Check sheet for the modelled part. Datum: model origin and axes. Units: mm. A direction names the side the tool comes from. Give positions to 0.01 mm unless a question says otherwise; leave off trailing zeros. Order: outer loops, then holes, each group sorted by start corner. A loop starts at its lowest first (then second) coordinate and runs counter-clockwise, first axis right, second up. Notation, with made-up numbers: (3.5, 45.5) -> (18.5, 45.5) arc R16 ccw to (18.5, 66.5) -> close; hole circle Ø10 at (60, -13). An arc over 180 degrees is marked (long way). Answer in a Markdown table with one row per item. Add a question column.
(1) Cross-section at B-B (z = 0). Record the cut outline in (x, y), then the cut area to 3 significant figures.
(2) Go/stop test with flat-tipped pins: pin 1 (2 mm diameter, centred on y = 20, z = -5, fed in from +X); pin 2 (3 mm diameter, centred on x = -19.5, z = -0.5, fed in from -Y); pin 3 (1.5 mm diameter, centred on y = 30.5, z = 3, fed in from +X). Record where each tip stops, or that it passes through.
(3) Cross-section at A-A (y = 4.5). Record the cut outline in (x, z).
(4) Thickness scan on L1, parallel to X at y = 13, z = 4.5; L2, parallel to Y at x = 23, z = 0. Record the ranges inside material, lowest first. Write a range as [from, to].
(5) Cross-section at D-D (y = 30). Record the cut outline in (x, z), then the cut area to 3 significant figures.
(6) Release check for a two-part mould opening along X. For faces 1 (the face through (0, 8, -12.7)), 2 (the face through (-25.4, 19, 0)), 3 (the face through (-2.86, 28.36, -5.22)) record: released by +X, released by -X, zero draft, split by the parting line, or undercut.
(7) Set-up check for faces 4 (the face through (-12.7, 8, 0)), 5 (the face through (-3, 31.4, 0)), 6 (the face through (22.269, 36.109, -6.827)): record each of +Z, -Z, +X, -X, +Y, -Y from which the full face is reachable in a straight line by a thin tool's end or side.
(8) Cross-section at C-C (x = 16.5). Record the cut outline in (y, z).
```python
from build123d import *

# Parameters (mm, degrees)
SKETCH2_W           = 50.8
SKETCH2_H           = 50.8
BOSS_EXTRUDE1_DEPTH = 50.8
SKETCH3_W           = 25.4
SKETCH3_H           = 25.4
SKETCH3_W_2         = 22.352
SKETCH3_H_2         = 22.352
CUT_EXTRUDE1_DEPTH  = 15.24
CUT_EXTRUDE2_DEPTH  = 51.8
SKETCH5_R           = 12.7
CUT_EXTRUDE3_DEPTH  = 6.35


with BuildPart() as part:
    # Sketch2 → Boss-Extrude1 (new body)
    with BuildSketch(Plane(origin=(0, 0, 0), x_dir=(1, 0, 0), z_dir=(0, 1, 0))):
        Rectangle(SKETCH2_W, SKETCH2_H)
    extrude(amount=BOSS_EXTRUDE1_DEPTH)

    # Sketch3 → Cut-Extrude1 (cut)
    with BuildSketch(Plane.XZ):
        Rectangle(SKETCH3_W, SKETCH3_H)
        Rectangle(SKETCH3_W_2, SKETCH3_H_2, mode=Mode.SUBTRACT)
    extrude(amount=-CUT_EXTRUDE1_DEPTH, mode=Mode.SUBTRACT)

    # Sketch4 → Cut-Extrude2 (cut, through all)
    with BuildSketch(Plane(origin=(25.4, 0, 0), x_dir=(0, 0, -1), z_dir=(1, 0, 0))):
        Polygon((6.92820323, 25.4), (3.464101615, 31.4), (-3.464101615, 31.4), (-6.92820323, 25.4), (-3.464101615, 19.4), (3.464101615, 19.4), align=None)
    extrude(amount=-CUT_EXTRUDE2_DEPTH, mode=Mode.SUBTRACT)

    # Sketch5 → Cut-Extrude3 (cut)
    with BuildSketch(Plane(origin=(25.4, 0, 0), x_dir=(0, 0, -1), z_dir=(1, 0, 0))):
        with Locations((0, 25.4)):
            Circle(SKETCH5_R)
    extrude(amount=-CUT_EXTRUDE3_DEPTH, mode=Mode.SUBTRACT)


solid = part.part
```
Answer below:
| question | item | result |
|---|---|---|
| 1 | outline | (-25.4, 0) -> (-12.7, 0) -> (-12.7, 15.24) -> (-11.18, 15.24) -> (-11.18, 0) -> (11.18, 0) -> (11.18, 15.24) -> (12.7, 15.24) -> (12.7, 0) -> (25.4, 0) -> (25.4, 12.7) -> (19.05, 12.7) -> (19.05, 19.4) -> (-25.4, 19.4) -> close; (-25.4, 31.4) -> (19.05, 31.4) -> (19.05, 38.1) -> (25.4, 38.1) -> (25.4, 50.8) -> (-25.4, 50.8) -> close |
| 1 | area | 1,840 mm² |
| 2 | pin 1 | stops at x = 19.05 |
| 2 | pin 2 | stops at y = 0 |
| 2 | pin 3 | passes through |
| 3 | outline | (-25.4, -25.4) -> (25.4, -25.4) -> (25.4, 25.4) -> (-25.4, 25.4) -> close; (-11.18, -11.18) -> (11.18, -11.18) -> (11.18, 11.18) -> (-11.18, 11.18) -> close; hole (-12.7, -12.7) -> (12.7, -12.7) -> (12.7, 12.7) -> (-12.7, 12.7) -> close |
| 4 | L1 | x = [-25.4, -12.7], [-11.18, 11.18], [12.7, 25.4] |
| 4 | L2 | y = [0, 12.7], [38.1, 50.8] |
| 5 | outline | (-25.4, -25.4) -> (25.4, -25.4) -> (25.4, -11.84) -> (19.05, -11.84) -> (19.05, -4.27) -> (-25.4, -4.27) -> close; (-25.4, 4.27) -> (19.05, 4.27) -> (19.05, 11.84) -> (25.4, 11.84) -> (25.4, 25.4) -> (-25.4, 25.4) -> close |
| 5 | area | 2,050 mm² |
| 6 | face 1 | undercut |
| 6 | face 2 | released by -X |
| 6 | face 3 | zero draft |
| 7 | face 4 | -Y |
| 7 | face 5 | +X, -X |
| 7 | face 6 | +X |
| 8 | outline | (0, -25.4) -> (50.8, -25.4) -> (50.8, 25.4) -> (0, 25.4) -> close; hole (19.4, -3.46) -> (25.4, -6.93) -> (31.4, -3.46) -> (31.4, 3.46) -> (25.4, 6.93) -> (19.4, 3.46) -> close |
